Source: CAD feature listing. Evaluate the final solid. Frame: model axes, mm. A direction names the side the tool comes from. Coordinates: 2 decimals unless noted, no trailing zeros. Order: outer loops, then holes, each group sorted by start corner. A loop starts at its lowest first (then second) coordinate and runs counter-clockwise, first axis right, second up.
Item 1: Section D-D on z = -20. Return the cut outline in (x, y).
Item 2: Mould query, pull axis Y, two halves, no side actions, for faces 6 (the flat face through (20.25, 0, -12)), 7 (the flat face through (0, 12, 34.5)), 8 (the flat face through (0, 2.275, 32)). Classes: released by +Y, released by -Y, zero draft, split by the parting line, or undercut.
Item 3: Section C-C on y = 5.5. Return the cut outline in (x, z).
Item 4: Section A-A on x = 0. State how many separate pieces and enclosed holes the cut face has, then the cut area to 3 significant figures.
Item 5: Reachability of faces 1 (the flat face through (-6.23, 3, 17)), 2 (the cylindrical face through (21.26, -0.47, -9.25)), 3 (the cylindrical face through (-1.321, -17.634, 33.614)), 4 (the cylindrical face through (-8.59, -10.41, 2.9)), 5 (the cylindrical face through (20.278, 14.268, -23.648)) from +Z, -Z, +X, -X, +Y, -Y: full face, straight path, thin tool, end or side. Return the list, or none.
Item 6: Contact query for flat-ended pins moving along their axis: P1, Ø2.5, axis at x = 1.5, z = 33, coming from the +Y side (3 decimals); P2, Ø4.5, axis at x = 0, y = 13.5, coming from the -Z side; P3, Ø4, axis at y = 9.5, z = 5, coming from the -X side. Output: stop coordinate, or through.
Item 7: Ray query, line 1 (Z direction, x = 0, y = 3.75); line 2 (Z direction, x = 21, y = 0); line 3 (X direction, y = -4, z = 14). Return the intervals inside material, ascending.
from build123d import *

# Parameters (mm, degrees)
SKETCH4_W                = 12.46
SKETCH4_H                = 17.25
BOSS_EXTRUDE3_DEPTH      = 6
SKETCH8_R                = 12.546781182
SKETCH8_R_2              = 11.15
BOSS_EXTRUDE6_DEPTH      = 8.3
BOSS_EXTRUDE6_DEPTH_BACK = 17.25
BOSS_EXTRUDE4_DEPTH      = 17.25
SKETCH6_R                = 0.75
CUT_EXTRUDE1_DEPTH       = 5
CHAMFER1_SIZE            = 0.5
CHAMFER1_SIZE2           = 0.866025404
SKETCH10_W               = 12.46
SKETCH10_H               = 23.7
CUT_EXTRUDE3_DEPTH       = 17.25
BOSS_EXTRUDE7_DEPTH      = 8.3
BOSS_EXTRUDE9_DEPTH      = 10
SKETCH20_R               = 11.15
SKETCH20_R_2             = 7.15
BOSS_EXTRUDE11_DEPTH     = 8.3
SKETCH21_R               = 10.15
SKETCH21_R_2             = 7.15
CUT_EXTRUDE7_DEPTH       = 1.3
SKETCH11_W               = 10
SKETCH11_H               = 2
CUT_EXTRUDE4_DEPTH       = 23.7
CUT_EXTRUDE8_REACH       = 37.55
SKETCH25_W               = 12.46
SKETCH25_H               = 6
BOSS_EXTRUDE10_DEPTH     = 35.55
SKETCH18_W               = 21.5
SKETCH18_H               = 11.438292938
CUT_EXTRUDE5_DEPTH       = 2
SKETCH19_R               = 3.5
CUT_EXTRUDE6_DEPTH       = 43.5
CUT_EXTRUDE6_DEPTH_BACK  = 3
FILLET1_R                = 10
SKETCH22_R               = 6.5
BOSS_EXTRUDE12_DEPTH     = 5
SKETCH23_R               = 5.85
BOSS_EXTRUDE13_DEPTH     = 5
FILLET2_R                = 1
BOSS_EXTRUDE14_DEPTH     = 2
CUT_EXTRUDE9_REACH       = 46.5
SKETCH27_R               = 0.75
CUT_EXTRUDE10_DEPTH      = 36.55
SKETCH29_R               = 2.1
SKETCH29_R_2             = 3.2
CUT_EXTRUDE11_DEPTH      = 7
FILLET3_R                = 1
SKETCH31_W               = 10
SKETCH31_H               = 35.55
BOSS_EXTRUDE15_DEPTH     = 3


with BuildPart() as part:
    # Sketch4 → Boss-Extrude3 (new body)
    with BuildSketch(Plane.XY):
        with Locations((0, -1.35)):
            Rectangle(SKETCH4_W, SKETCH4_H)
    extrude(amount=BOSS_EXTRUDE3_DEPTH)



with BuildPart() as body_2:
    # Sketch8 → Boss-Extrude6 (new body, two sides)
    with BuildSketch(Plane(origin=(0, -9.975, 0), x_dir=(-1, 0, 0), z_dir=(0, -1, 0))) as boss_extrude6_sk:
        with Locations((0, -23.55)):
            Circle(SKETCH8_R)
        with Locations((0, -23.55)):
            Circle(SKETCH8_R_2, mode=Mode.SUBTRACT)
    extrude(amount=BOSS_EXTRUDE6_DEPTH)
    extrude(boss_extrude6_sk.sketch, amount=-BOSS_EXTRUDE6_DEPTH_BACK)


with BuildPart() as part_1:
    add(part.part)

    add(body_2.part)  # Boss-Extrude4 merges body 2
    # Sketch5 → Boss-Extrude4 (add)
    with BuildSketch(Plane(origin=(0, 7.275, 0), x_dir=(1, 0, 0), z_dir=(0, 1, 0))):
        with BuildLine():
            Line((12.546781182, -23.55), (12.546781182, 0))
            Line((12.546781182, 0), (6.23, 0))
            Line((6.23, 0), (6.23, -29.7))
            Line((6.23, -29.7), (-6.23, -29.7))
            Line((-6.23, -29.7), (-6.23, 0))
            Line((-6.23, 0), (-12.546781182, 0))
            Line((-12.546781182, 0), (-12.546781182, -23.55))
            ThreePointArc((-12.546781182, -23.55), (0, -36.096781182), (12.546781182, -23.55))
        make_face()
    extrude(amount=-BOSS_EXTRUDE4_DEPTH)

    # Sketch6 → Cut-Extrude1 (cut)
    with BuildSketch(Plane(origin=(0, 7.275, 0), x_dir=(1, 0, 0), z_dir=(0, 1, 0))):
        with Locations((0, -3.6)):
            Circle(SKETCH6_R)
        with Locations((0, -32.1)):
            Circle(SKETCH6_R)
    extrude(amount=-CUT_EXTRUDE1_DEPTH, mode=Mode.SUBTRACT)

    # Chamfer1
    chamfer1_edges = [part_1.edges().sort_by_distance(p)[0] for p in [
        (-0.75, 7.275, 3.6),
        (-0.75, 7.275, 32.1),
    ]]
    chamfer1_side = [part_1.faces().sort_by_distance(p)[0] for p in [
        (0, 7.275, 35.657160381),
    ]]
    chamfer(chamfer1_edges, length=CHAMFER1_SIZE, length2=CHAMFER1_SIZE2, reference=chamfer1_side[0])

    # Sketch10 → Cut-Extrude3 (cut)
    with BuildSketch(Plane(origin=(0, 7.275, 0), x_dir=(1, 0, 0), z_dir=(0, 1, 0))):
        with Locations((0, -17.85)):
            Rectangle(SKETCH10_W, SKETCH10_H)
    extrude(amount=-CUT_EXTRUDE3_DEPTH, mode=Mode.SUBTRACT)

    # Sketch13 → Boss-Extrude7 (add)
    with BuildSketch(Plane.XZ.offset(18.275)):
        with BuildLine():
            Line((-12.546781182, 23.55), (-12.546781182, 0))
            Line((-12.546781182, 0), (12.546781182, 0))
            Line((12.546781182, 0), (12.546781182, 23.55))
            ThreePointArc((12.546781182, 23.55), (0, 11.003218818), (-12.546781182, 23.55))
        make_face()
    extrude(amount=-BOSS_EXTRUDE7_DEPTH)

    # Sketch15 → Boss-Extrude9 (add)
    with BuildSketch(Plane(origin=(0, 7.275, 0), x_dir=(1, 0, 0), z_dir=(0, 1, 0))):
        with BuildLine():
            Line((-12.546781182, 0), (12.546781182, 0))
            Line((12.546781182, 0), (12.546781182, -23.55))
            ThreePointArc((12.546781182, -23.55), (0, -36.096781182), (-12.546781182, -23.55))
            Line((-12.546781182, -23.55), (-12.546781182, 0))
        make_face()
        with BuildLine():
            Line((-6.23, -0.8), (6.23, -0.8))
            Line((6.23, -0.8), (6.23, -33))
            ThreePointArc((6.23, -33), (5.790660172, -34.060660172), (4.73, -34.5))
            Line((4.73, -34.5), (-4.73, -34.5))
            ThreePointArc((-4.73, -34.5), (-5.790660172, -34.060660172), (-6.23, -33))
            Line((-6.23, -33), (-6.23, -0.8))
        make_face(mode=Mode.SUBTRACT)
    extrude(amount=BOSS_EXTRUDE9_DEPTH)

    # Sketch20 → Boss-Extrude11 (add)
    with BuildSketch(Plane.XZ.offset(18.275)):
        with Locations((0, 23.55)):
            Circle(SKETCH20_R)
        with Locations((0, 23.55)):
            Circle(SKETCH20_R_2, mode=Mode.SUBTRACT)
    extrude(amount=-BOSS_EXTRUDE11_DEPTH)

    # Sketch21 → Cut-Extrude7 (cut)
    with BuildSketch(Plane.XZ.offset(18.275)):
        with Locations((0, 23.55)):
            Circle(SKETCH21_R)
        with Locations((0, 23.55)):
            Circle(SKETCH21_R_2, mode=Mode.SUBTRACT)
    extrude(amount=-CUT_EXTRUDE7_DEPTH, mode=Mode.SUBTRACT)

    # Sketch11 → Cut-Extrude4 (cut)
    with BuildSketch(Plane.XY.offset(29.7)):
        with Locations((0, -10.975)):
            Rectangle(SKETCH11_W, SKETCH11_H)
    extrude(amount=-CUT_EXTRUDE4_DEPTH, mode=Mode.SUBTRACT)

    # Sketch25 → Cut-Extrude8 (cut, up to next)
    with BuildSketch(Plane.XZ.offset(18.275), mode=Mode.PRIVATE) as cut_extrude8_sk1:
        with Locations((0, 9)):
            Rectangle(SKETCH25_W, SKETCH25_H)
    cut_extrude8_tool1 = extrude(cut_extrude8_sk1.sketch, amount=-CUT_EXTRUDE8_REACH, mode=Mode.PRIVATE) & part_1.part
    add(cut_extrude8_tool1.solids().sort_by_distance((0, -18.275, 9))[0], mode=Mode.SUBTRACT)

    # Sketch17 → Boss-Extrude10 (add)
    with BuildSketch(Plane(origin=(0, 17.275, 0), x_dir=(1, 0, 0), z_dir=(0, 1, 0))):
        Polygon((22.25, 26.5), (22.25, 0), (-22.25, 0), (-22.25, 26.5), (-18.25, 26.5), (-18.25, 5), (18.25, 5), (18.25, 26.5), align=None)
    extrude(amount=-BOSS_EXTRUDE10_DEPTH)

    # Sketch18 → Cut-Extrude5 (cut)
    with BuildSketch(Plane.ZY.offset(-18.25)):
        with Locations((-15.75, -0.5)):
            Rectangle(SKETCH18_W, SKETCH18_H)
    extrude(amount=-CUT_EXTRUDE5_DEPTH, mode=Mode.SUBTRACT)

    # Sketch19 → Cut-Extrude6 (cut, two sides)
    with BuildSketch(Plane.ZY.offset(-20.25)) as cut_extrude6_sk:
        with Locations((-20, -0.5)):
            Circle(SKETCH19_R)
    extrude(amount=CUT_EXTRUDE6_DEPTH, mode=Mode.SUBTRACT)
    extrude(cut_extrude6_sk.sketch, amount=-CUT_EXTRUDE6_DEPTH_BACK, mode=Mode.SUBTRACT)

    # Fillet1
    fillet1_edges = [part_1.edges().sort_by_distance(p)[0] for p in [
        (20.25, 17.275, -26.5),
        (-20.25, 17.275, -26.5),
        (-20.25, -18.275, -26.5),
        (20.25, -18.275, -26.5),
    ]]
    fillet(fillet1_edges, radius=FILLET1_R)

    # Sketch22 → Boss-Extrude12 (add)
    with BuildSketch(Plane.ZY.offset(22.25)):
        with Locations((-20, -0.5)):
            Circle(SKETCH22_R)
    extrude(amount=-BOSS_EXTRUDE12_DEPTH)

    # Sketch23 → Boss-Extrude13 (add)
    with BuildSketch(Plane(origin=(-17.25, 0, 0), x_dir=(0, 0, -1), z_dir=(1, 0, 0))):
        with Locations((20, -0.5)):
            Circle(SKETCH23_R)
    extrude(amount=BOSS_EXTRUDE13_DEPTH)

    # Fillet2
    fillet2_edges = [part_1.edges().sort_by_distance(p)[0] for p in [
        (-12.25, -0.5, -14.15),
    ]]
    fillet(fillet2_edges, radius=FILLET2_R)

    # Sketch26 → Boss-Extrude14 (add)
    with BuildSketch(Plane.ZY.offset(-20.25)):
        Polygon((-5, 2), (-20, 2.6585), (-26.5, 2.94385), (-26.5, 5.219146469), (-5, 5.219146469), align=None)
        Polygon((-20, -3.6585), (-5, -3), (-5, -6.219146469), (-26.5, -6.219146469), (-26.5, -3.94385), align=None)
    extrude(amount=BOSS_EXTRUDE14_DEPTH)

    # Sketch27 → Cut-Extrude9 (cut, up to next)
    with BuildSketch(Plane(origin=(22.25, 0, 0), x_dir=(0, 0, -1), z_dir=(1, 0, 0)), mode=Mode.PRIVATE) as cut_extrude9_sk1:
        with Locations((10, -0.5)):
            Circle(SKETCH27_R)
    cut_extrude9_tool1 = extrude(cut_extrude9_sk1.sketch, amount=-CUT_EXTRUDE9_REACH, mode=Mode.PRIVATE) & part_1.part
    add(cut_extrude9_tool1.solids().sort_by_distance((22.25, -0.5, -10))[0], mode=Mode.SUBTRACT)
    # Sketch27 → Cut-Extrude9 (cut, up to next)
    with BuildSketch(Plane(origin=(22.25, 0, 0), x_dir=(0, 0, -1), z_dir=(1, 0, 0)), mode=Mode.PRIVATE) as cut_extrude9_sk2:
        with Locations((7.5, -0.5)):
            Circle(SKETCH27_R)
    cut_extrude9_tool2 = extrude(cut_extrude9_sk2.sketch, amount=-CUT_EXTRUDE9_REACH, mode=Mode.PRIVATE) & part_1.part
    add(cut_extrude9_tool2.solids().sort_by_distance((22.25, -0.5, -7.5))[0], mode=Mode.SUBTRACT)
    # Sketch27 → Cut-Extrude9 (cut, up to next)
    with BuildSketch(Plane(origin=(22.25, 0, 0), x_dir=(0, 0, -1), z_dir=(1, 0, 0)), mode=Mode.PRIVATE) as cut_extrude9_sk3:
        with Locations((13, -0.5)):
            Circle(SKETCH27_R)
    cut_extrude9_tool3 = extrude(cut_extrude9_sk3.sketch, amount=-CUT_EXTRUDE9_REACH, mode=Mode.PRIVATE) & part_1.part
    add(cut_extrude9_tool3.solids().sort_by_distance((22.25, -0.5, -13))[0], mode=Mode.SUBTRACT)

    # Sketch28 → Cut-Extrude10 (cut, through all)
    with BuildSketch(Plane.XZ.offset(18.275)):
        Polygon((-12.546781182, 23.55), (-12.546781182, -11.553408701), (-1.720894485, -11.553408701), (-1.720894485, -30.302101254), (-26.809724616, -30.302101254), (-26.809724616, 23.55), align=None)
    extrude(amount=-CUT_EXTRUDE10_DEPTH, mode=Mode.SUBTRACT)

    # Sketch29 → Cut-Extrude11 (cut)
    with BuildSketch(Plane.ZY.offset(12.546781182)):
        with Locations((5, 9.5)):
            Circle(SKETCH29_R)
        with Locations((5, -10.5)):
            Circle(SKETCH29_R)
        with Locations((5, -0.5)):
            Circle(SKETCH29_R_2)
    extrude(amount=-CUT_EXTRUDE11_DEPTH, mode=Mode.SUBTRACT)

    # Fillet3
    fillet3_edges = [part_1.edges().sort_by_distance(p)[0] for p in [
        (-12.546781182, 9.5, 2.9),
        (-12.546781182, -10.5, 2.9),
    ]]
    fillet(fillet3_edges, radius=FILLET3_R)

    # Sketch31 → Boss-Extrude15 (add)
    with BuildSketch(Plane(origin=(12.546781182, 0, 0), x_dir=(0, 0, -1), z_dir=(1, 0, 0))):
        with Locations((-5, -0.5)):
            Rectangle(SKETCH31_W, SKETCH31_H)
    extrude(amount=BOSS_EXTRUDE15_DEPTH)


solid = part_1.part
Answer list:
1. outline: (18.25, -17.64) - (22.25, -17.64) - (22.25, -4) - (20.25, -4) - (20.25, -3.66) - (18.25, -3.66) - close; (18.25, 2.66) - (20.25, 2.66) - (20.25, 3) - (22.25, 3) - (22.25, 16.64) - (18.25, 16.64) - close
2. face 6: undercut
2. face 7: zero draft
2. face 8: released by +Y
3. outline: (-12.55, -5) - (18.25, -5) - (18.25, -26.5) - (22.25, -26.5) - (22.25, 0) - (15.55, 0) - (15.55, 10) - (12.55, 10) - (12.55, 23.55) arc R12.55 ccw to (-12.55, 23.55) - close; hole (-6.23, 6) - (6.23, 6) - (6.23, 29.7) - (-6.23, 29.7) - close; hole circle Ø1.5 at (0, 3.6); hole circle Ø1.5 at (0, 32.1)
4. separate pieces: 3
4. enclosed holes: 0
4. area: 514 mm2
5. face 1: +Y
5. face 2: +X, -X
5. face 3: -Y
5. face 4: -X
5. face 5: -Z, +X, -X, +Y
6. P1: stops at y = 7.275
6. P2: stops at z = -5
6. P3: stops at x = 6.23
7. line 1: z = -5 to 2.85, 4.35 to 6, 29.7 to 31.35, 32.85 to 36.1
7. line 2: z = -26.5 to -23.46, -16.54 to -13.56, -12.44 to -10.56, -9.44 to -8.06, -6.94 to 0
7. line 3: x = -12.55 to -6.23, 6.23 to 12.55
